For this review, use the dimensioned drawing (mm, ordinates from the lowest corner) and the shaded views. A direction names the side the tool comes from. Coordinates: 2 decimals unless noted, no trailing zeros. Write each loop counter-clockwise with the first axis right and the second up, starting at its lowest first coordinate (ties: lowest second). Pieces come first, ordered by that corner, then holes. Notation, with made-up numbers: (28.25, 67) - (52.25, 67) arc R20 cw to (52.25, 92) - close; hole circle Ø7 at (42, 59). An arc over 180 degrees is marked (long way). Use one line per item in the form item = value. Start each with the question number.
1) Tool access review of the marked faces 4, 5, 6 and 7: name each direction out of +Z, -Z, +X, -X, +Y, -Y from which nothing blocks a thin tool from reaching the whole face with its end or side.
2) We need section C-C (z = 87.5). Give the boundary of the cut face in (x, y), plus the area to 3 significant figures.
3) Mouldability with a two-part tool opening along Y and no side actions: class the marked faces 1, 2 and 3 as pulls with the +Y half, pulls with the -Y half, needs draft (parallel to the pull), parting line crosses it, or undercut.
4) We need section A-A (x = 51). Give the boundary of the cut face in (y, z).
5) For L1, parallel to X at y = 60.5, z = 53.5; L2, parallel to Y at x = 36, z = 67; L3, parallel to Y at x = 47.5, z = 127.5, list the stretches that pass through material, from the lowest coordinate up. Write a range as from..to.
6) Insertion check: P1, Ø8, axis at y = 48.5, z = 30, coming from the -X side; P2, Ø20.5, axis at x = 39.5, z = 152.5, coming from the -Y side; P3, Ø8, axis at x = 18.5, z = 83, coming from the -Y side; P4, Ø21, axis at x = 94, y = 74.5, coming from the +Z side. Each pin has a flat end and moves straight along its axis. Give the tip position at first contact, or say it passes through.
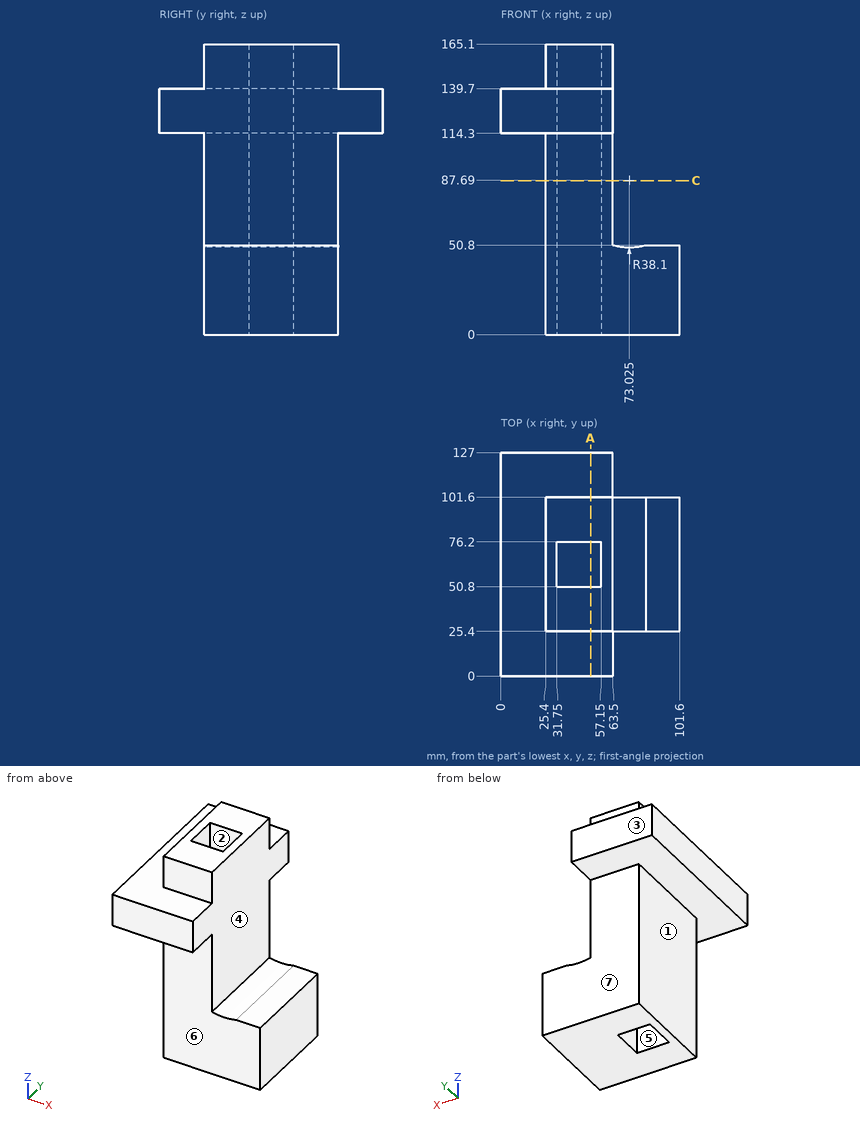
Determined:
q1.face_4 = +Z, +X, +Y, -Y
q1.face_5 = +Z, -Z
q1.face_6 = -Z, +X, -X, -Y
q1.face_7 = -Z, +X, -X, +Y
q2.outline = (25.4, 25.4) - (63.5, 25.4) - (63.5, 101.6) - (25.4, 101.6) - close; hole (31.75, 50.8) - (57.15, 50.8) - (57.15, 76.2) - (31.75, 76.2) - close
q2.area = 2,260 mm²
q3.face_1 = needs draft
q3.face_2 = undercut
q3.face_3 = pulls with the +Y half
q4.outline = (0, 114.3) - (25.4, 114.3) - (25.4, 0) - (50.8, 0) - (50.8, 165.1) - (25.4, 165.1) - (25.4, 139.7) - (0, 139.7) - close; (76.2, 0) - (101.6, 0) - (101.6, 114.3) - (127, 114.3) - (127, 139.7) - (101.6, 139.7) - (101.6, 165.1) - (76.2, 165.1) - close
q5.L1 = 25.4..31.75, 57.15..63.5
q5.L2 = 25.4..50.8, 76.2..101.6
q5.L3 = 0..50.8, 76.2..127
q6.P1 = 25.4
q6.P2 = 25.4
q6.P3 = through
q6.P4 = 50.8
